```python
from build123d import *

# Parameters (mm, degrees)
F0_W     = 82.651131
F0_H     = 60.990963
F1_DEPTH = 61.722
F2_R     = 7.971733
F4_D     = 12.7
F5_T     = -2.54


with BuildPart() as f1:
    # F0 (on Top) → F1 (new body)
    with BuildSketch(Plane.XY):
        with Locations((41.325565, -30.495482)):
            Rectangle(F0_W, F0_H)
    extrude(amount=F1_DEPTH)

    # F2
    f2_edges = [f1.edges().sort_by_distance(p)[0] for p in [
        (82.651131, -30.495482, 61.722),
    ]]
    fillet(f2_edges, radius=F2_R)

    # F4 (through all)
    with Locations(Plane.XY.offset(61.722)):
        with Locations((41.159108, -32.359846)):
            Hole(F4_D / 2)

    # F5
    f5_openings = [f1.faces().sort_by_distance(p)[0] for p in [
        (41.219566, -60.990963, 30.783051),
    ]]
    offset(amount=F5_T, openings=f5_openings)


solid = f1.part
```
Work out the finished part from the listing and answer in its coordinate system (mm). A direction names the side the tool comes from. Round coordinates to 2 decimals unless told otherwise and drop trailing zeros. Write each loop counter-clockwise with the first axis right and the second up, starting at its lowest first coordinate (ties: lowest second). Pieces come first, ordered by that corner, then holes.
1) Determine the mould class of faces 4 (the face through (80.111, -32, 28)), 5 (the face through (37, -23, 61.722)), 6 (the face through (82.651, -31, 26)), 7 (the face through (30, -31, 59.182)) for opening direction X: pulls with the +X half, pulls with the -X half, needs draft (parallel to the pull), parting line crosses it, or undercut.
2) A cutting plane is placed at C-C on z = 24.5. Determine the outline of the cut face in (x, y).
3) A cutting plane is placed at B-B on x = 36.5. Determine the outline of the cut face in (y, z), and give its area (3 significant figures).
4) A flat-ended cylindrical pin translates along its axis: P1, Ø8, axis at x = 20.5, y = -30, coming from the -Z side. Find the tip coordinate at first contact, or state that the pin passes through.
5) Consider probe 1 along Z at (x, y) = (60.5, -45); probe 2 along X at (y, z) = (-13.5, 15); probe 3 along X at (y, z) = (-29.5, 46). Determine where each line is inside the solid, lowest interval first.
6) Which of the six approach directions +Z, -Z, +X, -X, +Y, -Y give full straight-line access (tool end or side, diameter ignored) to faces 1 (the face through (43.086, -41.038, 30.465)), 2 (the face through (2.54, -32, 30)), 3 (the face through (0, -31, 30))?
7) A cutting plane is placed at D-D on y = -29. Determine the outline of the cut face in (x, z).
8) A cutting plane is placed at A-A on y = -8. Determine the outline of the cut face in (x, z).
Entries:
1. face 4: undercut
1. face 5: needs draft
1. face 6: pulls with the +X half
1. face 7: undercut
2. outline: (0, -60.99) - (2.54, -60.99) - (2.54, -2.54) - (80.11, -2.54) - (80.11, -60.99) - (82.65, -60.99) - (82.65, 0) - (0, 0) - close; circle Ø17.78 at (41.16, -32.36); hole circle Ø12.7 at (41.16, -32.36)
3. outline: (-60.99, 0) - (-36.67, 0) - (-36.67, 61.72) - (-60.99, 61.72) - (-60.99, 59.18) - (-39.93, 59.18) - (-39.93, 2.54) - (-60.99, 2.54) - close; (-28.05, 0) - (0, 0) - (0, 61.72) - (-28.05, 61.72) - close; hole (-24.79, 2.54) - (-2.54, 2.54) - (-2.54, 59.18) - (-24.79, 59.18) - close
3. area: 779 mm2
4. P1: stops at z = 0
5. probe 1: z = 0 to 2.54, 59.18 to 61.72
5. probe 2: x = 0 to 2.54, 80.11 to 82.65
5. probe 3: x = 0 to 2.54, 32.74 to 35.49, 46.83 to 49.58, 80.11 to 82.65
6. face 1: none
6. face 2: -Y
6. face 3: +Z, -Z, -X, +Y, -Y
7. outline: (0, 0) - (35.77, 0) - (35.77, 61.72) - (0, 61.72) - close; (46.55, 0) - (82.65, 0) - (82.65, 53.75) arc R7.97 ccw to (74.68, 61.72) - (46.55, 61.72) - close; hole (2.54, 2.54) - (32.93, 2.54) - (32.93, 59.18) - (2.54, 59.18) - close; hole (49.39, 2.54) - (80.11, 2.54) - (80.11, 53.75) arc R5.43 ccw to (74.68, 59.18) - (49.39, 59.18) - close
8. outline: (0, 0) - (82.65, 0) - (82.65, 53.75) arc R7.97 ccw to (74.68, 61.72) - (0, 61.72) - close; hole (2.54, 2.54) - (80.11, 2.54) - (80.11, 53.75) arc R5.43 ccw to (74.68, 59.18) - (2.54, 59.18) - close
